```python
from build123d import *

# Parameters (mm, degrees)
SKETCH1_W           = 56
SKETCH1_H           = 56
BOSS_EXTRUDE1_DEPTH = 7
SKETCH2_R           = 14.275
CUT_EXTRUDE1_DEPTH  = 8


with BuildPart() as part:
    # Sketch1 → Boss-Extrude1 (new body)
    with BuildSketch(Plane.XY):
        with Locations((28, 28)):
            Rectangle(SKETCH1_W, SKETCH1_H)
    extrude(amount=BOSS_EXTRUDE1_DEPTH)

    # Sketch2 → Cut-Extrude1 (cut, through all)
    with BuildSketch(Plane.XY.offset(7)):
        with Locations((28, 28)):
            Circle(SKETCH2_R)
        with BuildLine():
            Line((10.5, 48), (10.5, 8))
            ThreePointArc((10.5, 8), (8, 5.5), (5.5, 8))
            Line((5.5, 8), (5.5, 48))
            ThreePointArc((5.5, 48), (8, 50.5), (10.5, 48))
        make_face()
        with BuildLine():
            Line((50.5, 48), (50.5, 8))
            ThreePointArc((50.5, 8), (48, 5.5), (45.5, 8))
            Line((45.5, 8), (45.5, 48))
            ThreePointArc((45.5, 48), (48, 50.5), (50.5, 48))
        make_face()
    extrude(amount=-CUT_EXTRUDE1_DEPTH, mode=Mode.SUBTRACT)


solid = part.part
```
CAD build for the part. Positions are in the model's coordinates, mm. A direction names the side the tool comes from. Round coordinates to 2 decimals unless told otherwise and drop trailing zeros. Order: outer loops, then holes, each group sorted by start corner. A loop starts at its lowest first (then second) coordinate and runs counter-clockwise, first axis right, second up. Notation, with made-up numbers: (-5, 5.5) - (6, 5.5) arc R8 cw to (6, 17.5) - close; hole circle Ø5 at (-13.75, 61.25). An arc over 180 degrees is marked (long way). Answer in a Markdown table with one row per item. Add a question column.
(1) 3-axis set-ups, long thin cutter, end or side, ignore diameter. For faces 4 (the face through (48.1, 5.5, 3.5)), 5 (the face through (15, 35, 7)): which of +Z, -Z, +X, -X, +Y, -Y reach the whole face in a straight line?
(2) Band-saw the part on C-C on z = 3. List the corners of the cut face in (x, y) (3 decimals).
(3) Band-saw the part on D-D on x = 28. List the corners of the cut face in (y, z) (3 decimals).
(4) Band-saw the part on B-B on y = 28. List the corners of the cut face in (x, z) (3 decimals).
(5) Drop a flat-ended pin along its axis: pin 1 Ø4 at (x, y) = (50, 32.5) entering from -Z. Give the stop position or say it passes through.
(6) Mould opens along X. For faces 1 (the face through (15, 35, 0)), 2 (the face through (8.1, 5.5, 3.5)), 3 (the face through (56, 28, 3)) say: +X half, -X half, draft (parallel to the pull), parting line (faces both ways), or undercut.
(7) Probe L1, parallel to X at y = 27.5, z = 3.5; L2, parallel to Y at x = 28, z = 2.5 (3 decimals); L3, parallel to Y at x = 48, z = 6.5. List the from-to ranges inside material, lowest first. Write a range as [from, to].
(8) Band-saw the part on A-A on x = 48. List the corners of the cut face in (y, z), and give its area (3 significant figures).
Data:
| question | item | result |
|---|---|---|
| 1 | face 4 | +Z, -Z |
| 1 | face 5 | +Z, +X, -X, +Y, -Y |
| 2 | outline | (0, 0) - (56, 0) - (56, 56) - (0, 56) - close; hole (5.5, 8) arc R2.5 ccw to (10.5, 8) - (10.5, 48) arc R2.5 ccw to (5.5, 48) - close; hole circle Ø28.55 at (28, 28); hole (45.5, 8) arc R2.5 ccw to (50.5, 8) - (50.5, 48) arc R2.5 ccw to (45.5, 48) - close |
| 3 | outline | (0, 0) - (13.725, 0) - (13.725, 7) - (0, 7) - close; (42.275, 0) - (56, 0) - (56, 7) - (42.275, 7) - close |
| 4 | outline | (0, 0) - (5.5, 0) - (5.5, 7) - (0, 7) - close; (10.5, 0) - (13.725, 0) - (13.725, 7) - (10.5, 7) - close; (42.275, 0) - (45.5, 0) - (45.5, 7) - (42.275, 7) - close; (50.5, 0) - (56, 0) - (56, 7) - (50.5, 7) - close |
| 5 | pin 1 | stops at z = 0 |
| 6 | face 1 | draft |
| 6 | face 2 | undercut |
| 6 | face 3 | +X half |
| 7 | L1 | x = [0, 5.5], [10.5, 13.73], [42.27, 45.5], [50.5, 56] |
| 7 | L2 | y = [0, 13.725], [42.275, 56] |
| 7 | L3 | y = [0, 5.5], [50.5, 56] |
| 8 | outline | (0, 0) - (5.5, 0) - (5.5, 7) - (0, 7) - close; (50.5, 0) - (56, 0) - (56, 7) - (50.5, 7) - close |
| 8 | area | 77.0 mm^2 |
